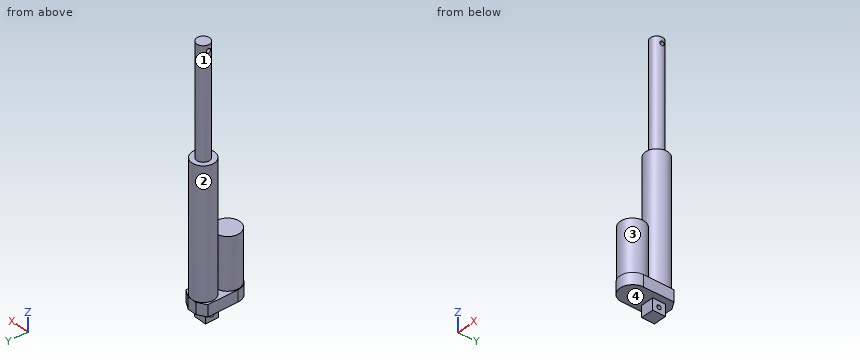
Autodesk Inventor part; units mm, degrees
ref_plane "YZ Plane" through (0, 0, 0) normal (1, 0, 0) x (0, 1, 0)
ref_plane "XZ Plane" through (0, 0, 0) normal (0, 1, 0) x (-1, 0, 0)
ref_plane "XY Plane" through (0, 0, 0) normal (0, 0, 1) x (1, 0, 0)
sketch "Sketch1" plane through (0, 0, 0) normal (0, 0, 1) x (1, 0, 0)
  line L0 (-10, -10) -> (10, -10)
  line L1 (10, -10) -> (10, 10)
  line L2 (10, 10) -> (-10, 10)
  line L3 (-10, 10) -> (-10, -10)
  line L4 (-10, -10) -> (10, 10) construction
  line L5 (10, -10) -> (-10, 10) construction
  line L6 (-20, 15) -> (-20, -32.5)
  line L7 (-20, 15) -> (-7.0096, 22.5)
  line L8 (-20, 15) -> (-5, 15) construction
  line L9 (-7.0096, 22.5) -> (7.0096, 22.5)
  line L10 (7.0096, 22.5) -> (20, 15)
  line L11 (20, 15) -> (20, -32.5)
  circle A0 centre (0, -32.5) radius 20 construction
  arc A1 (-20, -32.5) -> (20, -32.5) centre (0, -32.5) ccw
  point P0 (0, 0)
  point P1 (0, 22.5)
  point P2 (0, 10)
  dimension "d0" = 20
  dimension "d1" = 20
  dimension "d3" = 15
  dimension "d4" = 30
  dimension "d5" = 15
  dimension "d6" = 150
  dimension "d8" = 40
  dimension "d9" = 5
  dimension "d10" = 40
  dimension "d11" = 55
extrude "Extrusion1" add sketch "Sketch1" along normal blind 18
sketch "Sketch2" plane through (0, 0, 18) normal (0, 0, 1) x (1, 0, 0)
  line L0 (-10, -10) -> (-10, 10)
  line L1 (-10, 10) -> (10, 10)
  line L2 (10, 10) -> (10, -10)
  line L3 (10, -10) -> (-10, -10)
  line L4 (-20, 15) -> (-20, -32.5)
  arc A0 (-20, -32.5) -> (20, -32.5) centre (0, -32.5) ccw
  line L5 (20, -32.5) -> (20, 15)
  line L6 (20, 15) -> (7.0096, 22.5)
  line L7 (7.0096, 22.5) -> (-7.0096, 22.5)
  line L8 (-7.0096, 22.5) -> (-20, 15)
  point P0 (0, 0)
extrude "Extrusion2" add sketch "Sketch2" against normal blind 36 contours L0 L1 L2 L3
sketch "Sketch3" plane through (10, -10, 0) normal (1, 0, 0) x (0, 0, -1)
  circle A0 centre (9, 10) radius 3.25
  line L0 (0, 20) -> (18, 20)
  line L1 (0, 0) -> (0, 20)
  point P0 (0, 10)
  point P1 (9, 20)
  point P2 (0, 10)
  dimension "d16" = 6.5
extrude "Extrusion3" cut sketch "Sketch3" against normal through all
sketch "Sketch4" plane through (0, 0, 18) normal (0, 0, 1) x (1, 0, 0)
  circle A0 centre (0, 5) radius 17.5
  line L0 (7.0096, 22.5) -> (-7.0096, 22.5)
  point P0 (0, 0)
  point P1 (0, 22.5)
  dimension "d19" = 35
extrude "Extrusion4" add sketch "Sketch4" along normal blind 200
sketch "Sketch5" plane through (0, 0, 18) normal (0, 0, 1) x (1, 0, 0)
  circle A0 centre (0, -33) radius 19
  circle A1 centre (0, 5) radius 17.5
  point P0 (0, 0)
  dimension "d22" = 38
  dimension "d23" = 38
extrude "Extrusion5" add sketch "Sketch5" along normal blind 80 contours A0
sketch "Sketch10" plane through (0, 5, 218) normal (0, 0, 1) x (1, 0, 0)
  circle A0 centre (0, 0) radius 10
  circle A1 centre (0, 0) radius 17.5
  point P0 (0, -5)
  dimension "d32" = 20
extrude "Extrusion8" add sketch "Sketch10" along normal blind 152.4 contours A0
sketch "Sketch6" plane through (0, 5, 370.4) normal (0, 0, 1) x (1, 0, 0)
  circle A0 centre (0, 0) radius 17.5
  circle A1 centre (0, 0) radius 10
  point P0 (0, -5)
  dimension "d26" = 20
extrude "Extrusion6" add sketch "Sketch6" along normal blind 18 contours A1
sketch "Sketch8" plane through (0, 0, 0) normal (1, 0, 0) x (0, 1, 0)
  line L0 (15, 388.4) -> (-5, 388.4)
  line L1 (-5, 218) -> (15, 218)
  circle A0 centre (5, 379.4) radius 3.25
  line L2 (15, 388.4) -> (-5, 388.4)
  line L3 (15, 388.4) -> (15, 370.4)
  point P0 (0, 0)
  point P1 (5, 218)
  point P2 (15, 379.4)
  dimension "d29" = 6.5
  dimension "d35" = 18
extrude "Extrusion7" cut sketch "Sketch8" along normal through all both and the other way through all
properties part number "LinearActuator450" material "Steel, Carbon"
CAD build for the part. Positions are in the model's coordinates, mm. Face numbers are marked on the shaded views. Give positions to 0.01 mm unless a question says otherwise; leave off trailing zeros. Write each loop counter-clockwise with the first axis right and the second up, starting at its lowest first coordinate (ties: lowest second). Pieces come first, ordered by that corner, then holes. Notation, with made-up numbers: M 87.25,-10 L 129.25,-10 A20 ccw 129.25,28 Z; hole C -5,-24.5 d5. An arc over 180 degrees is marked long. Put each result on its own line as item: value. Start each with the question number.
(1) Band-saw the part on B-B, the plane y = -41. Write the cut outline in (x, z).
(2) Flat gauge pins, fed straight in: pin 1 Ø6 at (y, z) = (0, -9) entering from -X; pin 2 Ø3 at (x, z) = (10, 127.5) entering from +Y; pin 3 Ø2 at (x, y) = (7, -18.5) entering from +Z; pin 4 Ø5.5 at (x, z) = (-3, -10.5) entering from -Y. Where does each tip first touch, or does it go through?
(3) Band-saw the part on D-D, the plane z = 197.5. Write the cut outline in (x, y), and give its area (3 significant figures).
(4) Band-saw the part on C-C, the plane z = 250. Write the cut outline in (x, y), and give its area (3 significant figures).
(5) Mould opens along Y. For the marked faces 1, 2, 3 and 4 say: +Y half, -Y half, draft (parallel to the pull), parting line (faces both ways), or undercut.
(6) Band-saw the part on A-A, the plane z = 77.5. Write the cut outline in (x, y), and give its area (3 significant figures).
(7) Probe L1, parallel to Z at x = 2, y = 5; L2, parallel to Z at x = -8.5, y = -31.5; L3, parallel to X at y = -3, z = -1. List the from-to ranges inside material, lowest first.
Response values:
1. outline: M -18.1,0 L 18.1,0 L 18.1,18 L 17.23,18 L 17.23,98 L -17.23,98 L -17.23,18 L -18.1,18 Z
2. pin 1: passes through
2. pin 2: stops at y = 20.3
2. pin 3: stops at z = 98
2. pin 4: stops at y = -10
3. outline: C 0,5 d35
3. area: 962 mm2
4. outline: C 0,5 d20
4. area: 314 mm2
5. face 1: parting line
5. face 2: undercut
5. face 3: undercut
5. face 4: draft
6. outline: C 0,-33 d38; C 0,5 d35
6. area: 2,100 mm2
7. L1: z = -18 to 376.15, 382.65 to 388.4
7. L2: z = 0 to 98
7. L3: x = -10 to 10
